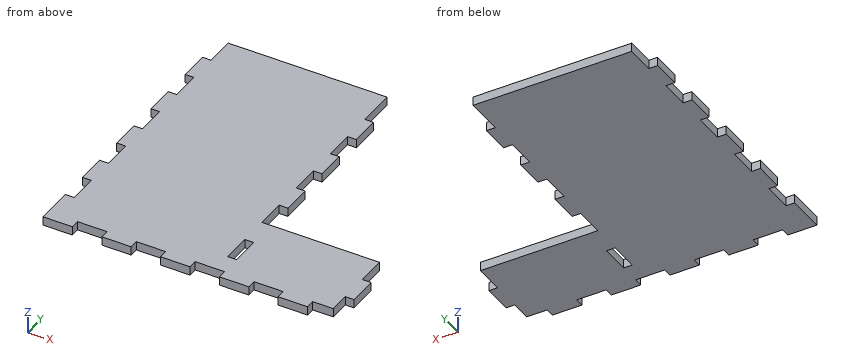
```python
from build123d import *

# Parameters (mm, degrees)
BOSS_EXTRUDE1_DEPTH = 6
SKETCH2_W           = 20
SKETCH2_H           = 6
CUT_EXTRUDE1_DEPTH  = 7
LPATTERN1_COUNT     = 5
LPATTERN1_PITCH     = 40
SKETCH3_W           = 6
SKETCH3_H           = 20
CUT_EXTRUDE2_DEPTH  = 7
LPATTERN2_COUNT     = 5
LPATTERN2_PITCH     = 40
SKETCH4_W           = 6
SKETCH4_H           = 6
CUT_EXTRUDE3_DEPTH  = 10
SKETCH5_W           = 6
SKETCH5_H           = 20
CUT_EXTRUDE4_DEPTH  = 10
LPATTERN3_COUNT     = 2
LPATTERN3_PITCH     = 40
SKETCH7_W           = 6
SKETCH7_H           = 20
CUT_EXTRUDE5_DEPTH  = 10
LPATTERN4_COUNT     = 5
LPATTERN4_PITCH     = 40


with BuildPart() as part:
    # Sketch1 → Boss-Extrude1 (new body)
    with BuildSketch(Plane.XY):
        Polygon((-17.330934256, 199.427419355), (102.669065744, 199.427419355), (102.669065744, 53.427419355), (182.669065744, 53.427419355), (182.669065744, -6.572580645), (102.669065744, -6.572580645), (-17.330934256, -6.572580645), align=None)
    extrude(amount=BOSS_EXTRUDE1_DEPTH)

    # Sketch2 → Cut-Extrude1 (cut, through all)
    with BuildSketch(Plane.XY.offset(6)):
        with Locations((12.669065744, -3.572580645)):
            Rectangle(SKETCH2_W, SKETCH2_H)
    cut_extrude1 = extrude(amount=-CUT_EXTRUDE1_DEPTH, mode=Mode.SUBTRACT)

    # LPattern1: Cut-Extrude1 ×5
    with Locations(*[(i * LPATTERN1_PITCH, 0, 0) for i in range(1, LPATTERN1_COUNT)]):
        add(cut_extrude1, mode=Mode.SUBTRACT)

    # Sketch3 → Cut-Extrude2 (cut, through all)
    with BuildSketch(Plane.XY):
        with Locations((99.669065744, 23.427419355)):
            Rectangle(SKETCH3_W, SKETCH3_H)
    cut_extrude2 = extrude(amount=CUT_EXTRUDE2_DEPTH, mode=Mode.SUBTRACT)

    # LPattern2: Cut-Extrude2 ×5
    with Locations(*[(0, i * LPATTERN2_PITCH, 0) for i in range(1, LPATTERN2_COUNT)]):
        add(cut_extrude2, mode=Mode.SUBTRACT)

    # Sketch4 → Cut-Extrude3 (cut)
    with BuildSketch(Plane.XY.offset(6)):
        with Locations((99.669065744, 196.427419355)):
            Rectangle(SKETCH4_W, SKETCH4_H)
    extrude(amount=-CUT_EXTRUDE3_DEPTH, mode=Mode.SUBTRACT)

    # Sketch5 → Cut-Extrude4 (cut)
    with BuildSketch(Plane.XY.offset(6)):
        with Locations((179.669065744, 43.427419355)):
            Rectangle(SKETCH5_W, SKETCH5_H)
    cut_extrude4 = extrude(amount=-CUT_EXTRUDE4_DEPTH, mode=Mode.SUBTRACT)

    # LPattern3: Cut-Extrude4 ×2
    with Locations(*[(0, -i * LPATTERN3_PITCH, 0) for i in range(1, LPATTERN3_COUNT)]):
        add(cut_extrude4, mode=Mode.SUBTRACT)

    # Sketch7 → Cut-Extrude5 (cut)
    with BuildSketch(Plane.XY.offset(6)):
        with Locations((-14.330934256, 189.427419355)):
            Rectangle(SKETCH7_W, SKETCH7_H)
    cut_extrude5 = extrude(amount=-CUT_EXTRUDE5_DEPTH, mode=Mode.SUBTRACT)

    # LPattern4: Cut-Extrude5 ×5
    with Locations(*[(0, -i * LPATTERN4_PITCH, 0) for i in range(1, LPATTERN4_COUNT)]):
        add(cut_extrude5, mode=Mode.SUBTRACT)


solid = part.part
```
Can you work these out from the model? Positions are in its coordinate system, mm. Coordinates: 2 decimals unless noted, no trailing zeros. Loops run counter-clockwise (first coordinate to the right, second up) from the corner with the lowest first, then second, coordinate; pieces in that order, holes last. Notation, with made-up numbers: (56, 53.25) -> (104, 53.25) arc R34 cw to (104, 83.25) -> close; hole circle Ø9 at (-2, -28.5). An arc over 180 degrees is marked (long way). Put each result on its own line as item: value. Start each with the question number.
Q1. I want a section at B-B (y = 51). Write out the boundary of the cut face in (x, z).
Q2. If I drill on line 1 (X direction, y = 26.5, z = 5.6); line 2 (Y direction, x = 149.5, z = 1.85); line 3 (X direction, y = 61, z = 2.25), over which ranges is the centre line in solid material (lowest first)? Write a range as [from, to].
Q3. I want a section at A-A (x = 146.5). Write out the boundary of the cut face in (y, z).
Q4. I'm going to push flat-ended pins straight in: P1, Ø1.8, axis at y = -4.5, z = 3, coming from the +X side; P2, Ø1.5, axis at y = 165.5, z = 2, coming from the +X side; P3, Ø1.8, axis at y = 106.5, z = 2.5, coming from the +X side. Where does each tip first touch, or does it pass through?
Taken from the geometry:
1. outline: (-17.33, 0) -> (176.67, 0) -> (176.67, 6) -> (-17.33, 6) -> close
2. line 1: x = [-11.33, 96.67], [102.67, 182.67]
2. line 2: y = [-6.57, 53.43]
2. line 3: x = [-11.33, 96.67]
3. outline: (-6.57, 0) -> (53.43, 0) -> (53.43, 6) -> (-6.57, 6) -> close
4. P1: stops at x = 162.67
4. P2: stops at x = 102.67
4. P3: stops at x = 96.67
